from build123d import *

# Parameters (mm, degrees)
F0_W     = 91.437164
F0_H     = 117.438275
F1_DEPTH = 76.2
F2_T     = -2.54
F3_W     = 86.357164
F3_H     = 6.434369
F4_DEPTH = 78.74


with BuildPart() as f1:
    # F0 (on Front) → F1 (new body)
    with BuildSketch(Plane.XZ):
        with Locations((2e-06, -5.200221)):
            Rectangle(F0_W, F0_H)
    extrude(amount=F1_DEPTH)

    # F2
    f2_openings = [f1.faces().sort_by_distance(p)[0] for p in [
        (2e-06, -76.2, -5.20022),
    ]]
    offset(amount=F2_T, openings=f2_openings)

    # F3 (on face) → F4 (join)
    with BuildSketch(Plane.XZ.offset(2.54)):
        with Locations((2e-06, 29.374299)):
            Rectangle(F3_W, F3_H)
    extrude(amount=F4_DEPTH)


solid = f1.part
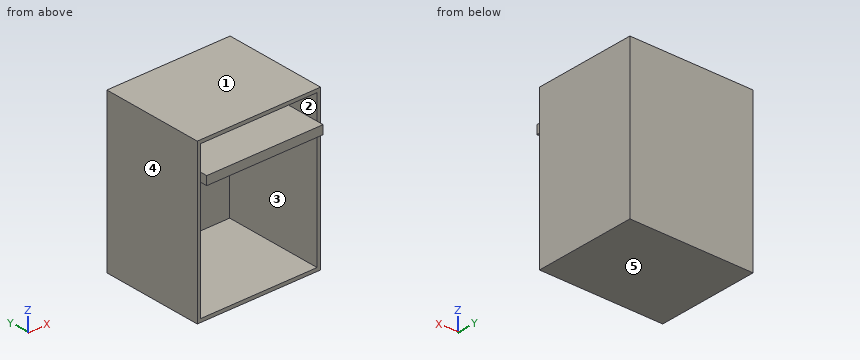
Model file for the job. Use its own axes, mm. Face numbers are marked on the shaded views. A direction names the side the tool comes from. Give positions to 0.01 mm unless a question says otherwise; leave off trailing zeros. Write each loop counter-clockwise with the first axis right and the second up, starting at its lowest first coordinate (ties: lowest second). Pieces come first, ordered by that corner, then holes. Notation, with made-up numbers: (14, -18.75) - (36, -18.75) arc R23 cw to (36, 9.25) - close; hole circle Ø5 at (12, -4). An arc over 180 degrees is marked (long way). Answer as CSV lines item,"result".
1. Band-saw the part on C-C (x = -12.5). Write the cut outline in (y, z), and give its area (3 significant figures).
Responses:
outline,"(-81.28, 26.16) - (-2.54, 26.16) - (-2.54, -61.38) - (-76.2, -61.38) - (-76.2, -63.92) - (0, -63.92) - (0, 53.52) - (-76.2, 53.52) - (-76.2, 50.98) - (-2.54, 50.98) - (-2.54, 32.59) - (-81.28, 32.59) - close"
area,"1,180 mm2"
2. Band-saw the part on A-A (y = -9.5). Write the cut outline in (x, z).
Responses:
outline,"(-45.72, -63.92) - (45.72, -63.92) - (45.72, 53.52) - (-45.72, 53.52) - close; hole (-43.18, -61.38) - (43.18, -61.38) - (43.18, 26.16) - (-43.18, 26.16) - close; hole (-43.18, 32.59) - (43.18, 32.59) - (43.18, 50.98) - (-43.18, 50.98) - close"
3. Drill centre lines: L1, parallel to Z at x = -8.5, y = -66.5; L2, parallel to X at y = -19, z = -41.5; L3, parallel to Y at x = -32, z = -19. Where is each one in solid material? Low to high. Write a range as [from, to].
Responses:
L1,"z = [-63.92, -61.38], [26.16, 32.59], [50.98, 53.52]"
L2,"x = [-45.72, -43.18], [43.18, 45.72]"
L3,"y = [-2.54, 0]"
4. Pin check, flat tips, straight feed: pin 1 (2.5 mm diameter, centred on y = -77.5, z = 28.5, fed in from -X); pin 2 (4 mm diameter, centred on x = 3, z = -5, fed in from +Y); pin 3 (5.5 mm diameter, centred on x = 9.5, z = 39.5, fed in from -Y); pin 4 (4 mm diameter, centred on y = -79.5, z = 30, fed in from +X). Stop position of each tip, or through.
Responses:
pin 1,"stops at x = -43.18"
pin 2,"stops at y = 0"
pin 3,"stops at y = -2.54"
pin 4,"stops at x = 43.18"
5. Band-saw the part on B-B (z = -37.5). Write the cut outline in (x, y).
Responses:
outline,"(-45.72, -76.2) - (-43.18, -76.2) - (-43.18, -2.54) - (43.18, -2.54) - (43.18, -76.2) - (45.72, -76.2) - (45.72, 0) - (-45.72, 0) - close"
6. 3-axis set-ups, long thin cutter, end or side, ignore diameter. For the marked faces 1 and 2: which of +Z, -Z, +X, -X, +Y, -Y reach the whole face in a straight line?
Responses:
face 1,"+Z, +X, -X, +Y, -Y"
face 2,"-Y"
7. Two-plate mould, pull along X, no slides. Class the marked faces 3, 4 and 5: +X half, -X half, draft (parallel to the pull), parting line (faces both ways), or undercut.
Responses:
face 3,"undercut"
face 4,"-X half"
face 5,"draft"
